Verification items for the finished model (mm, model axes). Face numbers are marked on the shaded views. A direction names the side the tool comes from. Round coordinates to 2 decimals unless told otherwise and drop trailing zeros. Loops run counter-clockwise (first coordinate to the right, second up) from the corner with the lowest first, then second, coordinate; pieces in that order, holes last. Notation, with made-up numbers: M -15.75,-24.75 L 42.25,-24.75 A27 ccw 42.25,4.25 Z; hole C -3,61.25 d10. An arc over 180 degrees is marked long. Write item = value, one per line. Start each with the question number.
from build123d import *

# Parameters (mm, degrees)
SKETCH1_W          = 139.7
SKETCH1_H          = 254
BASE_FLANGE1_DEPTH = 0.7
EDGE_FLANGE1_DEPTH = 139.7
SKETCH9_W          = 12.7
SKETCH9_H          = 23
TAB1_DEPTH         = 0.7
SKETCH12_W         = 12.7
SKETCH12_H         = 23
TAB2_DEPTH         = 0.7


# Sheet-metal steps are written as plain solids
with BuildPart() as part:
    # Sketch1 → Base-Flange1 (new body)
    with BuildSketch(Plane(origin=(0, 0, 0), x_dir=(1, 0, 0), z_dir=(0, 1, 0))):
        Rectangle(SKETCH1_W, SKETCH1_H)
    extrude(amount=-BASE_FLANGE1_DEPTH)

    # Edge-Flange1 section (across the edge) → Edge-Flange1 (add)
    with BuildSketch(Plane(origin=(69.85, 0, -128.8), x_dir=(0, 0, 1), z_dir=(-1, 0, 0))):
        with BuildLine():
            Line((-0.7, 1), (-0.7, 151.7))
            Line((-0.7, 151.7), (0, 151.7))
            Line((0, 151.7), (0, 1))
            ThreePointArc((0, 1), (0.292893219, 0.292893219), (1, 0))
            Line((1, 0), (1.8, 0))
            Line((1.8, 0), (1.8, -0.7))
            Line((1.8, -0.7), (1, -0.7))
            ThreePointArc((1, -0.7), (-0.202081528, -0.202081528), (-0.7, 1))
        make_face()
    extrude(amount=EDGE_FLANGE1_DEPTH)

    # Sketch9 → Tab1 (add)
    with BuildSketch(Plane(origin=(0, 0, 0), x_dir=(1, 0, 0), z_dir=(0, 1, 0))):
        with Locations((-63.5, -138.5)):
            Rectangle(SKETCH9_W, SKETCH9_H)
    extrude(amount=-TAB1_DEPTH)

    # Sketch12 → Tab2 (add)
    with BuildSketch(Plane(origin=(0, 0, 0), x_dir=(1, 0, 0), z_dir=(0, 1, 0))):
        with Locations((63.5, -138.5)):
            Rectangle(SKETCH12_W, SKETCH12_H)
    extrude(amount=-TAB2_DEPTH)


solid = part.part
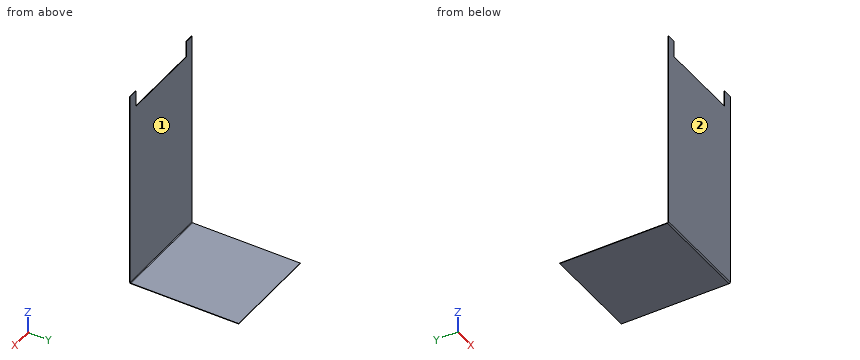
1. Section check C-C, the plane z = -37. Enter the section's corners in (x, y).
2. Gauge pin test, flat ends, axial feed: P1, Ø5, axis at x = -15, y = 111, coming from the +Z side; P2, Ø3, axis at x = 49, z = 120, coming from the +Y side. Record the tip position at first contact, or that the pin passes through.
3. Tool access check on the marked faces 1 and 2. Record the directions out of +Z, -Z, +X, -X, +Y, -Y that give a thin tool (end or side, any length) a straight path to the whole face; none if there is none.
4. Section check A-A, the plane x = 61. Enter the section's corners in (y, z).
5. Thickness scan on line 1 (Y direction, x = 32, z = -70); line 2 (Z direction, x = 16, y = 141.5). Record the ranges inside material, lowest first.
6. Section check B-B, the plane y = 76.5. Enter the section's corners in (x, z), and give its area (3 significant figures).
7. Section check D-D, the plane x = 38. Enter the section's corners in (y, z), and give its area (3 significant figures).
Computed values:
q1.outline = M -69.85,-0.7 L 69.85,-0.7 L 69.85,0 L -69.85,0 Z
q2.P1 = -128.8
q2.P2 = 0
q3.face_1 = +Z, +X, -X, +Y
q3.face_2 = +Z, -Z, +X, -X, -Y
q4.outline = M -0.7,-127.8 A1.7 ccw 1,-129.5 L 151.7,-129.5 L 151.7,-128.8 L 1,-128.8 A1 cw 0,-127.8 L 0,150 L -0.7,150 Z
q5.line_1 = -0.7 to 0
q5.line_2 = -129.5 to -128.8
q6.outline = M -69.85,-129.5 L 69.85,-129.5 L 69.85,-128.8 L -69.85,-128.8 Z
q6.area = 97.8 mm2
q7.outline = M -0.7,-127.8 A1.7 ccw 1,-129.5 L 151.7,-129.5 L 151.7,-128.8 L 1,-128.8 A1 cw 0,-127.8 L 0,127 L -0.7,127 Z
q7.area = 285 mm2
